Work out the finished part from the listing and answer in its coordinate system (mm). A direction names the side the tool comes from. Coordinates: 2 decimals unless noted, no trailing zeros. Order: outer loops, then holes, each group sorted by start corner. A loop starts at its lowest first (then second) coordinate and runs counter-clockwise, first axis right, second up. Notation, with made-up numbers: M -38,67 L -17,67 A20 ccw -17,106 Z; hole C 42.25,5 d1. An arc over 180 degrees is marked long. Answer in a Markdown table with one row per item. Add a question column.
Item 1: The part is cut by section A-A (z = 15). Write down the section's boundary in (x, y), then the cut area to 3 significant figures.
Item 2: The mould has two halves that part along Z. Classify faces 4 (the face through (-22.367, 3.042, -3.303)), 5 (the face through (0, 1, -60)), 6 (the face through (19.76, 3.04, -45.35)), 7 (the face through (-14, 4, -14)): released by +Z, released by -Z, zero draft, split by the parting line, or undercut.
Item 3: The part is cut by section B-B (z = -20.5). Write down the section's boundary in (x, y), then the cut area to 3 significant figures.
Item 4: The part is cut by section D-D (z = 33). Write down the section's boundary in (x, y), then the cut area to 3 significant figures.
Item 5: The part is cut by section C-C (y = 19.5). Write down the section's boundary in (x, z), then the cut area to 3 significant figures.
Item 6: Which of the six approach directions +Z, -Z, +X, -X, +Y, -Y give full straight-line access (tool end or side, diameter ignored) to faces 1 (the face through (23.86, 4.03, -46.9)), 2 (the face through (-17, 4, -47)), 3 (the face through (0, 1, -56.7))?
Item 7: Flat-ended cylindrical pins translate along their axes: pin 1 Ø3.5 at (x, z) = (-21, -3) entering from +Y; pin 2 Ø2.5 at (x, y) = (17.5, 3.5) entering from -Z; pin 3 Ø10 at (x, z) = (-15.5, 19.5) entering from +Y. Find the tip coordinate at first contact, or state that the pin passes through.
Item 8: Consider line 1 (X direction, y = 0.7, z = 15); line 2 (X direction, y = 2.25, z = -46); line 3 (X direction, y = 1.95, z = -3). Determine where each line is inside the solid, lowest interval first. Write a range as from..to.
from build123d import *

# Parameters (mm, degrees)
SKETCH_1_W             = 48
SKETCH_1_H             = 120
EXTRUDE_1_DEPTH        = 2
SKETCH_2_R             = 1.7
CUT_EXTRUDE_1_DEPTH    = 65.652919501
FILLET_1_R             = 3
SKETCH_3_R             = 1.8
CUT_EXTRUDE_2_DEPTH    = 2
SKETCH_4_W             = 10
SKETCH_4_H             = 2.6
EXTRUDE_2_DEPTH        = 22
RIB_6_REACH            = 76.967
SKETCH_5_WALL_W        = 175.020111274
SKETCH_5_WALL_H        = 2
SKETCH_6_R             = 2.2
CUT_EXTRUDE_3_DEPTH    = 76.463633626
FILLET_2_R             = 2
RIB_START              = -2
RIB_7_DEPTH            = 2
SKETCH_9_R             = 1.4
CUT_EXTRUDE_4_DEPTH    = 69.264192664
SKETCH_10_W            = 2
SKETCH_10_H            = 61.770189923
EXTRUDE_3_DEPTH        = 3
FILLET_3_R             = 2
CHAMFER_2_SIZE         = 3
HOLE_START             = -1
HOLE_WIZARD_M3_1_DEPTH = 4
EXTRUDE_START          = 4
SKETCH_14_R            = 3
SKETCH_14_R_2          = 1.4
EXTRUDE_4_DEPTH        = 4
SKETCH_15_W            = 4.171572875
SKETCH_15_H            = 2
EXTRUDE_5_DEPTH        = 3


with BuildPart() as part:
    # 草图1 → 凸台-拉伸1 (new body)
    with BuildSketch(Plane(origin=(0, 0, 0), x_dir=(1, 0, 0), z_dir=(0, 1, 0))):
        Rectangle(SKETCH_1_W, SKETCH_1_H)
    extrude(amount=EXTRUDE_1_DEPTH)

    # 草图2 → 切除-拉伸1 (cut, through all)
    with BuildSketch(Plane(origin=(0, 2, 0), x_dir=(1, 0, 0), z_dir=(0, 1, 0))):
        with Locations(Location((0, -55, 0), (0, 0, 90))):
            Circle(SKETCH_2_R)
        with BuildLine():
            Line((-1.5, 56.7), (1.5, 56.7))
            ThreePointArc((1.5, 56.7), (3.2, 55), (1.5, 53.3))
            Line((1.5, 53.3), (-1.5, 53.3))
            ThreePointArc((-1.5, 53.3), (-3.2, 55), (-1.5, 56.7))
        make_face()
    extrude(amount=-CUT_EXTRUDE_1_DEPTH, mode=Mode.SUBTRACT)

    # 圆角1
    fillet_1_edges = [part.edges().sort_by_distance(p)[0] for p in [
        (24, 1, 60),
        (-24, 1, 60),
        (-24, 1, -60),
        (24, 1, -60),
    ]]
    fillet(fillet_1_edges, radius=FILLET_1_R)

    # 草图3 → 切除-拉伸2 (cut)
    with BuildSketch(Plane(origin=(0, 0, 0), x_dir=(-1, 0, 0), z_dir=(0, -1, 0))):
        with Locations(Location((20, -15, 0), (0, 0, 90))):
            Circle(SKETCH_3_R)
        with Locations(Location((-20, -15, 0), (0, 0, 90))):
            Circle(SKETCH_3_R)
    extrude(amount=-CUT_EXTRUDE_2_DEPTH, mode=Mode.SUBTRACT)

    # 草图4 → 凸台-拉伸2 (add)
    with BuildSketch(Plane(origin=(0, 2, 0), x_dir=(1, 0, 0), z_dir=(0, 1, 0))):
        with Locations((19, -8.7)):
            Rectangle(SKETCH_4_W, SKETCH_4_H)
        with Locations((-19, -8.7)):
            Rectangle(SKETCH_4_W, SKETCH_4_H)
    extrude(amount=EXTRUDE_2_DEPTH)

    # 草图5 wall → 筋6 (add, up to next)
    with BuildSketch(Plane(origin=(14, 13, 3.9), x_dir=(0, -0.952925780013, -0.303203657277), z_dir=(0, -0.303203657277, 0.952925780013)), mode=Mode.PRIVATE) as rib_6_sk1:
        with Locations((0, 1)):
            Rectangle(SKETCH_5_WALL_W, SKETCH_5_WALL_H)
    rib_6_tool1 = extrude(rib_6_sk1.sketch, amount=RIB_6_REACH, mode=Mode.PRIVATE) - part.part
    rib_6 = rib_6_tool1.solids().sort_by_distance((14, 13, 3.9))[0]
    add(rib_6)

    # 镜向1: 筋6 across plane
    add(rib_6.mirror(Plane(origin=(0, 0, 0), x_dir=(0, 0, 1), z_dir=(1, 0, 0))))

    # 草图6 → 切除-拉伸3 (cut, through all)
    with BuildSketch(Plane(origin=(0, 0, 7.4), x_dir=(-1, 0, 0), z_dir=(0, 0, -1))):
        with Locations((-21, 19.5)):
            Circle(SKETCH_6_R)
        with Locations((21, 19.5)):
            Circle(SKETCH_6_R)
    extrude(amount=-CUT_EXTRUDE_3_DEPTH, mode=Mode.SUBTRACT)

    # 圆角2
    fillet_2_edges = [part.edges().sort_by_distance(p)[0] for p in [
        (24, 24, 8.7),
        (-24, 24, 8.7),
    ]]
    fillet(fillet_2_edges, radius=FILLET_2_R)

    # 筋7: read off the stored shape, not the designer's step
    # 筋7 outline → 筋7 (add)
    with BuildSketch(Plane(origin=(24, 0, 0), x_dir=(0, 0, -1), z_dir=(1, 0, 0)).offset(RIB_START)):
        Polygon((-3.4, 2), (-7.4, 14.571428571), (-7.4, 2), align=None)
    rib_7 = extrude(amount=RIB_7_DEPTH)

    # 镜向2: 筋7 across plane
    add(rib_7.mirror(Plane(origin=(0, 0, 0), x_dir=(0, 0, 1), z_dir=(1, 0, 0))))

    # 草图9 → 切除-拉伸4 (cut, through all)
    with BuildSketch(Plane(origin=(0, 2, 0), x_dir=(1, 0, 0), z_dir=(0, 1, 0))):
        with Locations(Location((-21, 46, 0), (0, 0, 270))):
            Circle(SKETCH_9_R)
        with Locations(Location((21, 46, 0), (0, 0, 270))):
            Circle(SKETCH_9_R)
        with Locations(Location((21, 3, 0), (0, 0, 270))):
            Circle(SKETCH_9_R)
        with Locations(Location((-21, 3, 0), (0, 0, 270))):
            Circle(SKETCH_9_R)
    extrude(amount=-CUT_EXTRUDE_4_DEPTH, mode=Mode.SUBTRACT)

    # 草图10 → 凸台-拉伸3 (add)
    with BuildSketch(Plane(origin=(0, 2, 0), x_dir=(1, 0, 0), z_dir=(0, 1, 0))):
        with Locations((-15, 29.114905039)):
            Rectangle(SKETCH_10_W, SKETCH_10_H)
        with Locations((15, 29.114905039)):
            Rectangle(SKETCH_10_W, SKETCH_10_H)
    extrude(amount=EXTRUDE_3_DEPTH)

    # 圆角3
    fillet_3_edges = [part.edges().sort_by_distance(p)[0] for p in [
        (-15, 5, 1.354545455),
        (15, 5, 1.354545455),
    ]]
    fillet(fillet_3_edges, radius=FILLET_3_R)

    # 倒角2
    chamfer_2_edges = [part.edges().sort_by_distance(p)[0] for p in [
        (15, 5, -60),
        (-15, 5, -60),
    ]]
    chamfer(chamfer_2_edges, length=CHAMFER_2_SIZE)

    # M3 十字槽沉头木螺钉的锥形沉头孔1: read off the stored shape, not the designer's step
    # M3 十字槽沉头木螺钉的锥形沉头孔1 outline → M3 十字槽沉头木螺钉的锥形沉头孔1 (cut)
    with BuildSketch(Plane(origin=(0, 0, 0), x_dir=(1, 0, 0), z_dir=(0, 1, 0)).offset(HOLE_START)):
        with BuildLine():
            Line((0, -56.7), (1.5, -56.7))
            ThreePointArc((1.5, -56.7), (3.2, -55), (1.5, -53.3))
            Line((1.5, -53.3), (0, -53.3))
            ThreePointArc((0, -53.3), (1.7, -55), (0, -56.7))
        make_face()
        with BuildLine():
            Line((-1.5, -56.7), (0, -56.7))
            ThreePointArc((0, -56.7), (-1.7, -55), (0, -53.3))
            Line((0, -53.3), (-1.5, -53.3))
            ThreePointArc((-1.5, -53.3), (-3.2, -55), (-1.5, -56.7))
        make_face()
    extrude(amount=HOLE_WIZARD_M3_1_DEPTH, mode=Mode.SUBTRACT)

    # Hole Wizard M3 _1 2: loft between two sections, ruled curve by curve
    hole_wizard_m3_1_2_from = [
        Edge.make_three_point_arc((1.5, 0.4, 56.7), (2.702081528, 0.4, 56.202081528), (3.2, 0.4, 55)),
        Edge.make_three_point_arc((3.2, 0.4, 55), (2.702081528, 0.4, 53.797918472), (1.5, 0.4, 53.3)),
        Edge.make_three_point_arc((-1.5, 0.4, 53.3), (-2.702081528, 0.4, 53.797918472), (-3.2, 0.4, 55)),
        Edge.make_three_point_arc((-3.2, 0.4, 55), (-2.702081528, 0.4, 56.202081528), (-1.5, 0.4, 56.7)),
        Edge.make_line((1.5, 0.4, 53.3), (-1.5, 0.4, 53.3)),
        Edge.make_line((1.5, 0.4, 56.7), (-1.5, 0.4, 56.7)),
    ]
    hole_wizard_m3_1_2_to = [
        Edge.make_three_point_arc((1.5, 2, 58.3), (3.833452378, 2, 57.333452378), (4.8, 2, 55)),
        Edge.make_three_point_arc((4.8, 2, 55), (3.833452378, 2, 52.666547622), (1.5, 2, 51.7)),
        Edge.make_three_point_arc((-1.5, 2, 51.7), (-3.833452378, 2, 52.666547622), (-4.8, 2, 55)),
        Edge.make_three_point_arc((-4.8, 2, 55), (-3.833452378, 2, 57.333452378), (-1.5, 2, 58.3)),
        Edge.make_line((1.5, 2, 51.7), (-1.5, 2, 51.7)),
        Edge.make_line((1.5, 2, 58.3), (-1.5, 2, 58.3)),
    ]
    hole_wizard_m3_1_2 = Solid(Shell([*[Face.make_surface_from_curves(hole_wizard_m3_1_2_from[k], hole_wizard_m3_1_2_to[k]) for k in range(6)], Face(Wire(hole_wizard_m3_1_2_from)), Face(Wire(hole_wizard_m3_1_2_to))]))
    add(hole_wizard_m3_1_2, mode=Mode.SUBTRACT)

    # 草图14 → 凸台-拉伸4 (add)
    # profile 1 of 4: a face of its own
    with BuildSketch(Plane(origin=(0, 2, 0), x_dir=(1, 0, 0), z_dir=(0, 1, 0)).offset(EXTRUDE_START)):
        with Locations(Location((-21, 46, 0), (0, 0, 180))):
            Circle(SKETCH_14_R)
        with Locations(Location((-21, 46, 0), (0, 0, 270))):
            Circle(SKETCH_14_R_2, mode=Mode.SUBTRACT)
    # profile 2 of 4: a face of its own
    with BuildSketch(Plane(origin=(0, 2, 0), x_dir=(1, 0, 0), z_dir=(0, 1, 0)).offset(EXTRUDE_START)):
        with Locations(Location((-21, 3, 0), (0, 0, 180))):
            Circle(SKETCH_14_R)
        with Locations(Location((-21, 3, 0), (0, 0, 270))):
            Circle(SKETCH_14_R_2, mode=Mode.SUBTRACT)
    # profile 3 of 4: a face of its own
    with BuildSketch(Plane(origin=(0, 2, 0), x_dir=(1, 0, 0), z_dir=(0, 1, 0)).offset(EXTRUDE_START)):
        with Locations((21, 46)):
            Circle(SKETCH_14_R)
        with Locations(Location((21, 46, 0), (0, 0, 270))):
            Circle(SKETCH_14_R_2, mode=Mode.SUBTRACT)
    # profile 4 of 4: a face of its own
    with BuildSketch(Plane(origin=(0, 2, 0), x_dir=(1, 0, 0), z_dir=(0, 1, 0)).offset(EXTRUDE_START)):
        with Locations((21, 3)):
            Circle(SKETCH_14_R)
        with Locations(Location((21, 3, 0), (0, 0, 270))):
            Circle(SKETCH_14_R_2, mode=Mode.SUBTRACT)
    extrude(amount=-EXTRUDE_4_DEPTH)

    # 草图15 → 凸台-拉伸5 (add)
    with BuildSketch(Plane(origin=(0, 5, 0), x_dir=(1, 0, 0), z_dir=(0, 1, 0))):
        with Locations((-16.085786438, 46)):
            Rectangle(SKETCH_15_W, SKETCH_15_H)
        with Locations((-16.085786438, 3)):
            Rectangle(SKETCH_15_W, SKETCH_15_H)
        with Locations((16.085786438, 3)):
            Rectangle(SKETCH_15_W, SKETCH_15_H)
        with Locations((16.085786438, 46)):
            Rectangle(SKETCH_15_W, SKETCH_15_H)
    extrude(amount=-EXTRUDE_5_DEPTH)


solid = part.part
Reply:
| question | item | result |
|---|---|---|
| 1 | outline | M -24,0 L -21.8,0 L -21.8,2 L -24,2 Z; M -18.2,0 L 18.2,0 L 18.2,2 L -18.2,2 Z; M 21.8,0 L 24,0 L 24,2 L 21.8,2 Z |
| 1 | area | 81.6 mm2 |
| 2 | face 4 | undercut |
| 2 | face 5 | released by -Z |
| 2 | face 6 | undercut |
| 2 | face 7 | zero draft |
| 3 | outline | M -24,0 L 24,0 L 24,2 L 16,2 L 16,5 L 14,5 L 14,2 L -14,2 L -14,5 L -16,5 L -16,2 L -24,2 Z |
| 3 | area | 108 mm2 |
| 4 | outline | M -24,0 L 24,0 L 24,2 L -24,2 Z |
| 4 | area | 96.0 mm2 |
| 5 | outline | M -24,7.4 L -23.2,7.4 L -23.2,10 L -24,10 Z; M -18.8,7.4 L -16,7.4 L -16,5.97 L -14,5.97 L -14,10 L -18.8,10 Z; M 14,5.97 L 16,5.97 L 16,7.4 L 18.8,7.4 L 18.8,10 L 14,10 Z; M 23.2,7.4 L 24,7.4 L 24,10 L 23.2,10 Z |
| 5 | area | 34.8 mm2 |
| 6 | face 1 | +Y |
| 6 | face 2 | -Z, +Y |
| 6 | face 3 | +Y, -Y |
| 7 | pin 1 | stops at y = 6 |
| 7 | pin 2 | stops at z = -47.98 |
| 7 | pin 3 | stops at y = 2 |
| 8 | line 1 | x = -24..-21.8, -18.2..18.2, 21.8..24 |
| 8 | line 2 | x = -24..-22.4, -19.6..-14, 14..19.6, 22.4..24 |
| 8 | line 3 | x = -24..-22.4, -19.6..19.6, 22.4..24 |
